```python
from build123d import *

# Parameters (mm, degrees)
SKETCH_1_R      = 2.5
EXTRUDE_1_DEPTH = 230
FILLET_1_R      = 1.5


with BuildPart() as part:
    # 草图1 → 凸台-拉伸1 (new body)
    with BuildSketch(Plane(origin=(0, 0, 0), x_dir=(1, 0, 0), z_dir=(0, 1, 0))):
        Polygon((3.9, 2.839339828), (3.9, -2.839339828), (6.560660172, -5.5), (8, -5.5), (8, -3.1), (9, -3.1), (9, -3.65), (10, -3.65), (10, -10), (3.65, -10), (3.65, -9), (3.1, -9), (3.1, -8), (5.5, -8), (5.5, -6.560660172), (2.839339828, -3.9), (-2.839339828, -3.9), (-5.5, -6.560660172), (-5.5, -8), (-3.1, -8), (-3.1, -9), (-3.65, -9), (-3.65, -10), (-10, -10), (-10, -3.65), (-9, -3.65), (-9, -3.1), (-8, -3.1), (-8, -5.5), (-6.560660172, -5.5), (-3.9, -2.839339828), (-3.9, 2.839339828), (-6.560660172, 5.5), (-8, 5.5), (-8, 3.1), (-9, 3.1), (-9, 3.65), (-10, 3.65), (-10, 10), (-3.65, 10), (-3.65, 9), (-3.1, 9), (-3.1, 8), (-5.5, 8), (-5.5, 6.560660172), (-2.839339828, 3.9), (2.839339828, 3.9), (5.5, 6.560660172), (5.5, 8), (3.1, 8), (3.1, 9), (3.65, 9), (3.65, 10), (10, 10), (10, 3.65), (9, 3.65), (9, 3.1), (8, 3.1), (8, 5.5), (6.560660172, 5.5), align=None)
        Circle(SKETCH_1_R, mode=Mode.SUBTRACT)
    extrude(amount=EXTRUDE_1_DEPTH)

    # 圆角1
    fillet_1_edges = [part.edges().sort_by_distance(p)[0] for p in [
        (-10, 115, 10),
        (-10, 115, -10),
        (10, 115, -10),
        (10, 115, 10),
    ]]
    fillet(fillet_1_edges, radius=FILLET_1_R)


solid = part.part
```
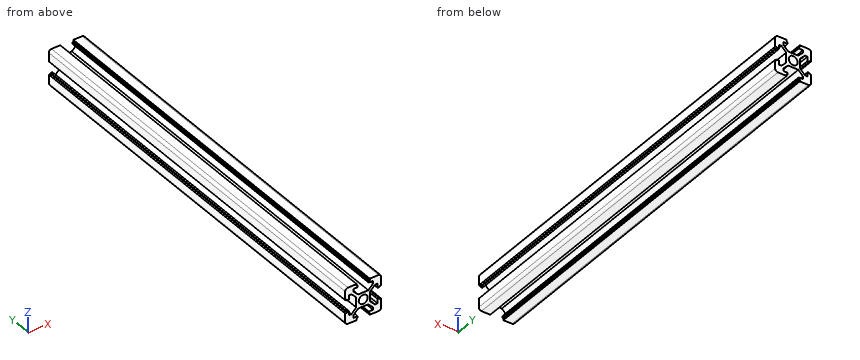
Can you work these out from the model? Positions are in its coordinate system, mm. Give positions to 0.01 mm unless a question says otherwise; leave off trailing zeros. Loops run counter-clockwise (first coordinate to the right, second up) from the corner with the lowest first, then second, coordinate; pieces in that order, holes last. Notation, with made-up numbers: M 87,84.25 L 121,84.25 A22 cw 121,108.25 Z; hole C 36,-22 d1. An arc over 180 degrees is marked long. Use CSV: the item, a comma, the result in double quotes. Start each with the question number.
1. If I drill on L1, parallel to Z at x = -8.75, y = 31.5; L2, parallel to X at y = 77, z = 0; L3, parallel to Z at x = -5.25, y = 40, over which ranges is the centre line in solid material (lowest first)?
2. Imagine slicing it at A-A, the plane x = 0. Write out the boundary of the cut face in (y, z), plus the area to 3 significant figures.
3. For P1, Ø1.5, axis at x = 2, z = -6, coming from the -Y side; P2, Ø0.5, axis at y = 89.5, z = 9.5, coming from the +X side; P3, Ø3, axis at x = -1, y = 60.5, coming from the -Z side; P4, Ø1.1, axis at x = -9.5, y = 98.5, coming from the -Z side, each with a flat end and sliding along its axis, tell me the tip position at first contact or that it passes through.
4. Imagine slicing it at B-B, the plane z = 0. Write out the boundary of the cut face in (x, y).
Response values:
1,L1,"-9.98 to -3.1, 3.1 to 9.98"
1,L2,"-3.9 to -2.5, 2.5 to 3.9"
1,L3,"-10 to -8, -6.31 to -4.19, 4.19 to 6.31, 8 to 10"
2,outline,"M 0,-3.9 L 230,-3.9 L 230,-2.5 L 0,-2.5 Z; M 0,2.5 L 230,2.5 L 230,3.9 L 0,3.9 Z"
2,area,"644 mm^2"
3,P1,"through"
3,P2,"x = 9.8"
3,P3,"z = -3.9"
3,P4,"z = -9.93"
4,outline,"M -3.9,0 L -2.5,0 L -2.5,230 L -3.9,230 Z; M 2.5,0 L 3.9,0 L 3.9,230 L 2.5,230 Z"
